from build123d import *

# Parameters (mm, degrees)
SKETCH2_R           = 15.875
SKETCH2_R_2         = 2.54
BOSS_EXTRUDE1_DEPTH = 3.175
FILLET1_R           = 2.54
SKETCH4_OUTSIDE_W   = 171.436
SKETCH4_OUTSIDE_H   = 82.536
SKETCH4_OUTSIDE_W_2 = 82.55
SKETCH4_OUTSIDE_H_2 = 50.8
CUT_EXTRUDE1_DEPTH  = 509.64451302
FILLET2_R           = 2.54


with BuildPart() as part:
    # Sketch2 → Boss-Extrude1 (new body)
    with BuildSketch(Plane.XY):
        Polygon((-508, 25.4), (-481.624580264, 25.4), (-457.99375, 25.4), (-431.8, 25.4), (-368.3, 25.4), (-368.3, -25.4), (-431.8, -25.4), (-457.99375, -25.4), (-481.624580264, -25.4), (-508, -25.4), align=None)
        with Locations((-469.9, 0)):
            Circle(SKETCH2_R, mode=Mode.SUBTRACT)
        with Locations((-495.3, 12.7)):
            Circle(SKETCH2_R_2, mode=Mode.SUBTRACT)
        with Locations((-495.3, -12.7)):
            Circle(SKETCH2_R_2, mode=Mode.SUBTRACT)
        with Locations((-444.5, -12.7)):
            Circle(SKETCH2_R_2, mode=Mode.SUBTRACT)
        with Locations((-431.8, -12.7)):
            Circle(SKETCH2_R_2, mode=Mode.SUBTRACT)
        with Locations((-419.1, -12.7)):
            Circle(SKETCH2_R_2, mode=Mode.SUBTRACT)
        with Locations((-419.1, 0)):
            Circle(SKETCH2_R_2, mode=Mode.SUBTRACT)
        with Locations((-431.8, 0)):
            Circle(SKETCH2_R_2, mode=Mode.SUBTRACT)
        with Locations((-431.8, 12.7)):
            Circle(SKETCH2_R_2, mode=Mode.SUBTRACT)
        with Locations((-419.1, 12.7)):
            Circle(SKETCH2_R_2, mode=Mode.SUBTRACT)
        with Locations((-444.5, 12.7)):
            Circle(SKETCH2_R_2, mode=Mode.SUBTRACT)
        with Locations((-406.4, 12.7)):
            Circle(SKETCH2_R_2, mode=Mode.SUBTRACT)
        with Locations((-406.4, 0)):
            Circle(SKETCH2_R_2, mode=Mode.SUBTRACT)
        with Locations((-406.4, -12.7)):
            Circle(SKETCH2_R_2, mode=Mode.SUBTRACT)
        with Locations((-393.7, 12.7)):
            Circle(SKETCH2_R_2, mode=Mode.SUBTRACT)
        with Locations((-393.7, 0)):
            Circle(SKETCH2_R_2, mode=Mode.SUBTRACT)
        with Locations((-393.7, -12.7)):
            Circle(SKETCH2_R_2, mode=Mode.SUBTRACT)
        with Locations((-381, 12.7)):
            Circle(SKETCH2_R_2, mode=Mode.SUBTRACT)
        with Locations((-381, 0)):
            Circle(SKETCH2_R_2, mode=Mode.SUBTRACT)
        with Locations((-381, -12.7)):
            Circle(SKETCH2_R_2, mode=Mode.SUBTRACT)
    extrude(amount=BOSS_EXTRUDE1_DEPTH)

    # Fillet1
    fillet1_edges = [part.edges().sort_by_distance(p)[0] for p in [
        (-508, 25.4, 1.5875),
        (-368.3, 25.4, 1.5875),
        (-368.3, -25.4, 1.5875),
        (-508, -25.4, 1.5875),
    ]]
    fillet(fillet1_edges, radius=FILLET1_R)

    # Sketch4 outside → Cut-Extrude1 (cut, through all)
    with BuildSketch(Plane.XY.offset(3.175)):
        with Locations((-438.15, 0)):
            Rectangle(SKETCH4_OUTSIDE_W, SKETCH4_OUTSIDE_H)
        with Locations((-466.725, 0)):
            Rectangle(SKETCH4_OUTSIDE_W_2, SKETCH4_OUTSIDE_H_2, mode=Mode.SUBTRACT)
    extrude(amount=-CUT_EXTRUDE1_DEPTH, mode=Mode.SUBTRACT)

    # Fillet2
    fillet2_edges = [part.edges().sort_by_distance(p)[0] for p in [
        (-425.45, 25.4, 1.5875),
        (-425.45, -25.4, 1.5875),
    ]]
    fillet(fillet2_edges, radius=FILLET2_R)


solid = part.part
Design review of the part built by this model. Coordinates are the model's own, in mm. Round coordinates to 2 decimals unless told otherwise and drop trailing zeros. Loops run counter-clockwise (first coordinate to the right, second up) from the corner with the lowest first, then second, coordinate; pieces in that order, holes last. Notation, with made-up numbers: M 87.5,-12.5 L 96.5,-12.5 A9 ccw 96.5,-4.5 Z; hole C 38.5,5.25 d4. An arc over 180 degrees is marked long. Answer as a JSON object with one key per item and string values.
Item 1: We need section B-B on x = -444.5. Give the boundary of the cut face in (y, z) (3 decimals).
Answer sheet:
{"outline": "M -25.4,0 L -15.24,0 L -15.24,3.175 L -25.4,3.175 Z; M -10.16,0 L 10.16,0 L 10.16,3.175 L -10.16,3.175 Z; M 15.24,0 L 25.4,0 L 25.4,3.175 L 15.24,3.175 Z"}
Item 2: We need section C-C on z = 1.95. State how many separate pieces and enclosed holes the cut face has, and give its area (3 significant figures).
Answer sheet:
{"separate pieces": "1", "enclosed holes": "8", "area": "3,250 mm^2"}
Item 3: We need section D-D on y = 8. Give the boundary of the cut face in (x, z) (3 decimals), and give its area (3 significant figures).
Answer sheet:
{"outline": "M -508,0 L -483.612,0 L -483.612,3.175 L -508,3.175 Z; M -456.188,0 L -425.45,0 L -425.45,3.175 L -456.188,3.175 Z", "area": "175 mm^2"}
Item 4: We need section A-A on y = 0. Give the boundary of the cut face in (x, z) (3 decimals).
Answer sheet:
{"outline": "M -508,0 L -485.775,0 L -485.775,3.175 L -508,3.175 Z; M -454.025,0 L -434.34,0 L -434.34,3.175 L -454.025,3.175 Z; M -429.26,0 L -425.45,0 L -425.45,3.175 L -429.26,3.175 Z"}
Item 5: Wall thickness on L1, parallel to Y at x = -431.8, z = 0.9; L2, parallel to Y at x = -444.5, z = 1.7; L3, parallel to Y at x = -469.9, z = 0.6 (3 decimals): over which ranges is each line inside the solid? List them lowest first. Write a range as from..to.
Answer sheet:
{"L1": "y = -25.4..-15.24, -10.16..-2.54, 2.54..10.16, 15.24..25.4", "L2": "y = -25.4..-15.24, -10.16..10.16, 15.24..25.4", "L3": "y = -25.4..-15.875, 15.875..25.4"}
